from build123d import *

# Parameters (mm, degrees)
EXTRUDE_1_DEPTH      = 12.5
EXTRUDE_1_DEPTH_BACK = 12.5
SKETCH_1_R           = 9.5
SKETCH_2_R           = 2.5
CUT_EXTRUDE_1_DEPTH  = 8
SKETCH_3_R           = 4
CUT_EXTRUDE_2_DEPTH  = 18
FILLET_1_R           = 0.5
FILLET_2_R           = 0.5


with BuildPart() as part:
    # 草图1 → 凸台-拉伸1 (new, two sides: drawn at the far end of the back side and taken through both)
    with BuildSketch(Plane.XY.offset(-EXTRUDE_1_DEPTH_BACK)):
        Circle(SKETCH_1_R)
    extrude(amount=EXTRUDE_1_DEPTH + EXTRUDE_1_DEPTH_BACK)

    # 草图2 → 切除-拉伸1 (cut)
    with BuildSketch(Plane.XY.offset(12.5)):
        Circle(SKETCH_2_R)
    extrude(amount=-CUT_EXTRUDE_1_DEPTH, mode=Mode.SUBTRACT)

    # 草图3 → 切除-拉伸2 (cut)
    with BuildSketch(Plane(origin=(0, 0, -12.5), x_dir=(-1, 0, 0), z_dir=(0, 0, -1))):
        Circle(SKETCH_3_R)
    extrude(amount=-CUT_EXTRUDE_2_DEPTH, mode=Mode.SUBTRACT)

    # 圆角1
    fillet_1_edges = [part.edges().sort_by_distance(p)[0] for p in [
        (-9.5, 0, -12.5),
    ]]
    fillet(fillet_1_edges, radius=FILLET_1_R)

    # 圆角2
    fillet_2_edges = [part.edges().sort_by_distance(p)[0] for p in [
        (-9.5, 0, 12.5),
    ]]
    fillet(fillet_2_edges, radius=FILLET_2_R)


solid = part.part
Part model, mm, in its own coordinate system. A direction names the side the tool comes from. Give positions to 0.01 mm unless a question says otherwise; leave off trailing zeros. Loops run counter-clockwise (first coordinate to the right, second up) from the corner with the lowest first, then second, coordinate; pieces in that order, holes last. Notation, with made-up numbers: M 0,84 L 42,84 A21 cw 42,107 Z; hole C -14.75,30 d10. An arc over 180 degrees is marked long. Put each result on its own line as item: value. Start each with the question number.
1) Saw through at C-C (z = 9.75). List the corners of the cut face in (x, y).
2) 3-axis set-ups, long thin cutter, end or side, ignore diameter. For faces 1 (the flat face through (-2, 2, 5.5)), 2 (the flat face through (2, -2, 12.5)): which of +Z, -Z, +X, -X, +Y, -Y reach the whole face in a straight line?
3) Saw through at D-D (z = 5). List the corners of the cut face in (x, y).
4) Probe probe 1 along Y at (x, z) = (0, 10.75); probe 2 along Y at (x, z) = (-0.25, 2); probe 3 along X at (y, z) = (1, 3.25). List the from-to ranges inside material, lowest first.
5) Flat gauge pins, fed straight in: pin 1 (1.5 mm diameter, centred on y = 3.5, z = -8.5, fed in from -X); pin 2 (4 mm diameter, centred on y = 6.5, z = -8.5, fed in from -X); pin 3 (6 mm diameter, centred on x = 0, y = 0, fed in from -Z); pin 4 (6.5 mm diameter, centred on x = -0.5, y = 2, fed in from -Z). Where does each tip first touch, or does it go through?
6) Saw through at A-A (y = 0). List the corners of the cut face in (x, z), then the cut area to 3 significant figures.
7) Pull direction Y, two halves, no side cores. Call faces 3 (the flat face through (4, -2, -12.5)), 4 (the cylindrical face through (4.38, -8.43, -0.17)), 5 (the cylindrical face through (0.867, -3.905, -3.626)): +Y half, -Y half, draft (parallel to the pull), parting line (faces both ways), or undercut.
Numbers:
1. outline: C 0,0 d19; hole C 0,0 d5
2. face 1: -Z
2. face 2: +Z, +X, -X, +Y, -Y
3. outline: C 0,0 d19; hole C 0,0 d8
4. probe 1: -9.5 to -2.5, 2.5 to 9.5
4. probe 2: -9.5 to -3.99, 3.99 to 9.5
4. probe 3: -9.45 to -3.87, 3.87 to 9.45
5. pin 1: x = -9.09
5. pin 2: x = -8.37
5. pin 3: z = 5.5
5. pin 4: z = -12.5
6. outline: M -9.5,-12 A0.5 ccw -9,-12.5 L -4,-12.5 L -4,5.5 L -2.5,5.5 L -2.5,12.5 L -9,12.5 A0.5 ccw -9.5,12 Z; M 2.5,5.5 L 4,5.5 L 4,-12.5 L 9,-12.5 A0.5 ccw 9.5,-12 L 9.5,12 A0.5 ccw 9,12.5 L 2.5,12.5 Z
6. area: 296 mm^2
7. face 3: draft
7. face 4: parting line
7. face 5: undercut
